```python
from build123d import *

# Parameters (mm, degrees)
SKETCH1_R           = 2
BOSS_EXTRUDE1_DEPTH = 3.3
SKETCH2_W           = 60
SKETCH2_H           = 3.3
BOSS_EXTRUDE2_DEPTH = 26
FILLET1_R           = 3
SKETCH4_R           = 1.5
SKETCH4_R_2         = 4.5
CUT_EXTRUDE1_DEPTH  = 18


with BuildPart() as part:
    # Sketch1 → Boss-Extrude1 (new body)
    with BuildSketch(Plane.XY):
        with BuildLine():
            Line((30, -17), (-30, -17))
            Line((-30, -17), (-30, 12))
            ThreePointArc((-30, 12), (-28.535533906, 15.535533906), (-25, 17))
            Line((-25, 17), (25, 17))
            ThreePointArc((25, 17), (28.535533906, 15.535533906), (30, 12))
            Line((30, 12), (30, -17))
        make_face()
        with Locations((-24.5, 5)):
            Circle(SKETCH1_R, mode=Mode.SUBTRACT)
        with Locations((24.5, 5)):
            Circle(SKETCH1_R, mode=Mode.SUBTRACT)
        with Locations((24.5, -5)):
            Circle(SKETCH1_R, mode=Mode.SUBTRACT)
        with Locations((-24.5, -5)):
            Circle(SKETCH1_R, mode=Mode.SUBTRACT)
        with Locations((-25, 12)):
            Circle(SKETCH1_R, mode=Mode.SUBTRACT)
        with Locations((25, 12)):
            Circle(SKETCH1_R, mode=Mode.SUBTRACT)
        with BuildLine():
            Line((-20.35, -4), (-20.35, -10.25))
            Line((-20.35, -10.25), (20.35, -10.25))
            Line((20.35, -10.25), (20.35, -4))
            ThreePointArc((20.35, -4), (20.935786438, -2.585786438), (22.35, -2))
            Line((22.35, -2), (26.5, -2))
            Line((26.5, -2), (26.5, 2))
            Line((26.5, 2), (22.35, 2))
            ThreePointArc((22.35, 2), (20.935786438, 2.585786438), (20.35, 4))
            Line((20.35, 4), (20.35, 10.25))
            Line((20.35, 10.25), (-20.35, 10.25))
            Line((-20.35, 10.25), (-20.35, 4))
            ThreePointArc((-20.35, 4), (-20.935786438, 2.585786438), (-22.35, 2))
            Line((-22.35, 2), (-26.5, 2))
            Line((-26.5, 2), (-26.5, -2))
            Line((-26.5, -2), (-22.35, -2))
            ThreePointArc((-22.35, -2), (-20.935786438, -2.585786438), (-20.35, -4))
        make_face(mode=Mode.SUBTRACT)
    boss_extrude1 = extrude(amount=BOSS_EXTRUDE1_DEPTH)

    # Sketch2 → Boss-Extrude2 (add)
    with BuildSketch(Plane.XY.offset(3.3)):
        with Locations((0, -15.35)):
            Rectangle(SKETCH2_W, SKETCH2_H)
    extrude(amount=-BOSS_EXTRUDE2_DEPTH)

    # Mirror1: Boss-Extrude1 across plane
    add(boss_extrude1.mirror(Plane.XY.offset(-11.35)))

    # Fillet1
    fillet1_edges = [part.edges().sort_by_distance(p)[0] for p in [
        (0, -13.7, -22.7),
        (0, -13.7, 0),
        (0, -17, -26),
        (0, -17, 3.3),
    ]]
    fillet(fillet1_edges, radius=FILLET1_R)

    # Sketch4 → Cut-Extrude1 (cut)
    with BuildSketch(Plane.XZ.offset(17)):
        with Locations((-22.778174593, -3.571825407)):
            Circle(SKETCH4_R)
        with Locations((-7.221825407, -3.571825407)):
            Circle(SKETCH4_R)
        with Locations((-7.221825407, -19.128174593)):
            Circle(SKETCH4_R)
        with Locations((-22.778174593, -19.128174593)):
            Circle(SKETCH4_R)
        with Locations((22.778174593, -19.128174593)):
            Circle(SKETCH4_R)
        with Locations((7.221825407, -19.128174593)):
            Circle(SKETCH4_R)
        with Locations((7.221825407, -3.571825407)):
            Circle(SKETCH4_R)
        with Locations((22.778174593, -3.571825407)):
            Circle(SKETCH4_R)
        with Locations((-15, -11.35)):
            Circle(SKETCH4_R_2)
        with Locations((15, -11.35)):
            Circle(SKETCH4_R_2)
    extrude(amount=-CUT_EXTRUDE1_DEPTH, mode=Mode.SUBTRACT)


solid = part.part
```
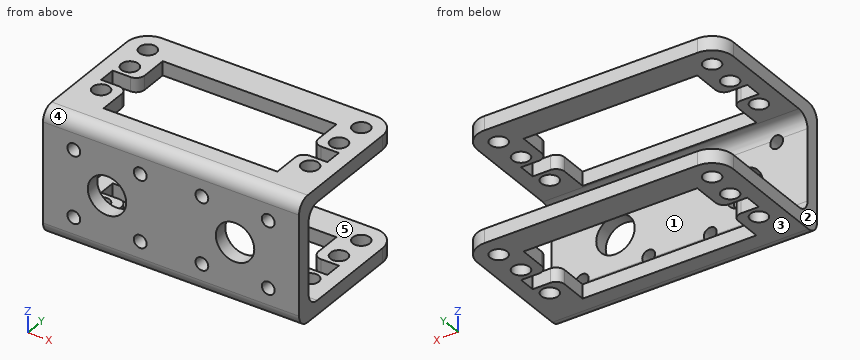
The listing builds one solid part. Answer for the finished solid, in the listing's coordinates (mm). Face numbers are marked on the shaded views. A direction names the side the tool comes from. Give positions to 0.01 mm unless a question says otherwise; leave off trailing zeros. Write each loop counter-clockwise with the first axis right and the second up, starting at its lowest first coordinate (ties: lowest second). Pieces come first, ordered by that corner, then holes. Notation, with made-up numbers: (47.5, -23.75) -> (68.5, -23.75) arc R15 ccw to (68.5, -5.75) -> close; hole circle Ø8 at (47.5, 60.25). An arc over 180 degrees is marked (long way). Write item = value, one per line. Start each with the question number.
1) The part is cut by section C-C, the plane x = 15. Determine the outline of the cut face in (y, z).
2) The part is cut by section D-D, the plane y = -5. Count the separate pieces of the cut face and the enclosed holes in it, and give its area (3 significant figures).
3) Determine the mould class of the marked faces 1, 2 and 3 for opening direction Z: +Z half, -Z half, draft (parallel to the pull), parting line (faces both ways), or undercut.
4) This flat-tipped pin is pushed along its axis until it touches: pin 1 (5 mm diameter, centred on x = 7.22, z = -19.13, fed in from +Y). Where does it stop, or does it pass through?
5) The part is cut by section A-A, the plane y = 1. Determine the outline of the cut face in (x, z), and give its area (3 significant figures).
6) Straight lines are drawn through the part: line 1 along Z through (x, y) = (-21.5, -9.5); line 2 along Y through (x, z) = (24.5, -24.5); line 3 along X through (y, z) = (13.5, -23.5). For each, find the intervals that lie inside material, in ascending order.
7) Which of the six approach directions +Z, -Z, +X, -X, +Y, -Y give full straight-line access (tool end or side, diameter ignored) to the marked faces 4 and 5?
8) The part is cut by section B-B, the plane z = -7.75. Determine the outline of the cut face in (x, y).
Solutions:
q1.outline = (-17, -23) arc R3 ccw to (-14, -26) -> (-10.25, -26) -> (-10.25, -22.7) -> (-10.7, -22.7) arc R3 cw to (-13.7, -19.7) -> (-13.7, -15.85) -> (-17, -15.85) -> close; (-17, -6.85) -> (-13.7, -6.85) -> (-13.7, -3) arc R3 cw to (-10.7, 0) -> (-10.25, 0) -> (-10.25, 3.3) -> (-14, 3.3) arc R3 ccw to (-17, 0.3) -> close; (10.25, -26) -> (17, -26) -> (17, -22.7) -> (10.25, -22.7) -> close; (10.25, 0) -> (17, 0) -> (17, 3.3) -> (10.25, 3.3) -> close
q2.separate_pieces = 8
q2.enclosed_holes = 0
q2.area = 74.6 mm²
q3.face_1 = undercut
q3.face_2 = draft
q3.face_3 = -Z half
q4.pin_1 = -13
q5.outline = (-30, -26) -> (-26.5, -26) -> (-26.5, -22.7) -> (-30, -22.7) -> close; (-30, 0) -> (-26.5, 0) -> (-26.5, 3.3) -> (-30, 3.3) -> close; (26.5, -26) -> (30, -26) -> (30, -22.7) -> (26.5, -22.7) -> close; (26.5, 0) -> (30, 0) -> (30, 3.3) -> (26.5, 3.3) -> close
q5.area = 46.2 mm²
q6.line_1 = -26 to -22.7, 0 to 3.3
q6.line_2 = -16.6 to -7, -3 to -2, 2 to 3, 7 to 10.06, 13.94 to 17
q6.line_3 = -29.77 to -26.32, -23.68 to 23.68, 26.32 to 29.77
q7.face_4 = +Z, +X, -X, -Y
q7.face_5 = +X, -X, +Y
q8.outline = (-30, -17) -> (-17.7, -17) -> (-17.7, -13.7) -> (-30, -13.7) -> close; (-12.3, -17) -> (12.3, -17) -> (12.3, -13.7) -> (-12.3, -13.7) -> close; (17.7, -17) -> (30, -17) -> (30, -13.7) -> (17.7, -13.7) -> close
